from build123d import *

# Parameters (mm, degrees)
EXTRUDE_1_DEPTH          = 2
EXTRUDE_3_DEPTH          = 2
SKETCH_5_W               = 7
SKETCH_5_H               = 7
SKETCH_5_R               = 1.25
EXTRUDE_4_DEPTH          = 7
SKETCH_6_W               = 7
SKETCH_6_H               = 7
SKETCH_6_R               = 1.25
EXTRUDE_5_DEPTH          = 7
CUT_EXTRUDE_1_DEPTH      = 7
CUT_EXTRUDE_1_DEPTH_BACK = 2


with BuildPart() as part:
    # Эскиз1 → Бобышка-Вытянуть1 (new body)
    with BuildSketch(Plane.XY):
        Polygon((-30, 20.5), (-28, 22.5), (4.828427125, 22.5), (12.328427125, 15), (28, 15), (30, 13), (30, -22.5), (-30, -22.5), align=None)
    extrude(amount=EXTRUDE_1_DEPTH)

    # Эскиз4 → Бобышка-Вытянуть3 (add)
    with BuildSketch(Plane(origin=(0, 0, 0), x_dir=(-1, 0, 0), z_dir=(0, 0, -1))):
        Polygon((-27.7, -20.2), (-27.7, 12.7), (-11.375735931, 12.7), (-3.875735931, 20.2), (27.7, 20.2), (27.7, -20.2), align=None)
        Polygon((-25.7, 10.7), (-10.547308807, 10.7), (-3.047308807, 18.2), (25.7, 18.2), (25.7, -18.2), (-25.7, -18.2), align=None, mode=Mode.SUBTRACT)
    extrude(amount=EXTRUDE_3_DEPTH)

    # Эскиз5 → Бобышка-Вытянуть4 (add)
    with BuildSketch(Plane(origin=(27.7, 0, 0), x_dir=(0, 0, -1), z_dir=(1, 0, 0))):
        with Locations((3.5, 9.2)):
            Rectangle(SKETCH_5_W, SKETCH_5_H)
        with Locations((3.5, 9.2)):
            Circle(SKETCH_5_R, mode=Mode.SUBTRACT)
    extrude(amount=-EXTRUDE_4_DEPTH)

    # Эскиз6 → Бобышка-Вытянуть5 (add)
    with BuildSketch(Plane.ZY.offset(27.7)):
        with Locations((-3.5, 16.7)):
            Rectangle(SKETCH_6_W, SKETCH_6_H)
        with Locations((-3.5, 16.7)):
            Circle(SKETCH_6_R, mode=Mode.SUBTRACT)
    extrude(amount=-EXTRUDE_5_DEPTH)

    # Эскиз7 → Вырез-Вытянуть1 (cut, two sides)
    with BuildSketch(Plane(origin=(0, 0, 0), x_dir=(-1, 0, 0), z_dir=(0, 0, -1))) as cut_extrude_1_sk:
        with BuildLine():
            Line((26.5, 7.555), (26.5, -7.525))
            ThreePointArc((26.5, -7.525), (23.5, -10.525), (20.5, -7.525))
            Line((20.5, -7.525), (20.5, 7.555))
            ThreePointArc((20.5, 7.555), (23.5, 10.555), (26.5, 7.555))
        make_face()
    extrude(amount=CUT_EXTRUDE_1_DEPTH, mode=Mode.SUBTRACT)
    extrude(cut_extrude_1_sk.sketch, amount=-CUT_EXTRUDE_1_DEPTH_BACK, mode=Mode.SUBTRACT)


solid = part.part
Part model, mm, in its own coordinate system. A direction names the side the tool comes from. Coordinates: 2 decimals unless noted, no trailing zeros. Loops run counter-clockwise (first coordinate to the right, second up) from the corner with the lowest first, then second, coordinate; pieces in that order, holes last. Notation, with made-up numbers: M 30,35 L 84,35 A24 cw 84,69 Z; hole C -36,-13 d8. An arc over 180 degrees is marked long. Use a Markdown table: item, result. Add a question column.
Q1. Cut at A-A (z = -3.5). Write the cut outline in (x, y), and give its area (3 significant figures).
Q2. Cut at B-B (y = 0.5). Write the cut outline in (x, z).
Q3. Mould opens along X. For faces 6 (the flat face through (-24, 17, -7)), 7 (the flat face through (30, -5, 1)), 8 (the cylindrical face through (-24.59, -10.32, 0.47)) say: +X half, -X half, draft (parallel to the pull), parting line (faces both ways), or undercut.
Q4. Cut at C-C (x = 13). Write the cut outline in (y, z).
Q5. Which spindle directions (+Z, -Z, +X, -X, +Y, -Y) get a long thin tool onto all of the face, cutting with end or side? Do faces 1 (the flat face through (0, 19, -2)), 2 (the flat face through (0, -22.5, 1)), 3 (the cylindrical face through (-24.464, 10.396, 0.472)), 4 (the flat face through (7.678, 16.398, -0.986)), 5 (the flat face through (24, 5.7, -3)). Say none if no direction does.
Q6. Cut at D-D (x = 25). Write the cut outline in (y, z), and give its area (3 significant figures).
Q7. Probe L1, parallel to Y at x = 22.25, z = -3.5; L2, parallel to X at y = 6.5, z = -0.5; L3, parallel to Y at x = 24.5, z = -1. List the from-to ranges inside material, lowest first.
Q8. Pin check, flat tips, straight feed: P1, Ø1, axis at x = 5.5, z = -3, coming from the -Y side; P2, Ø0.6, axis at x = 11.5, z = -1, coming from the -Y side; P3, Ø2, axis at x = 0, y = 1.5, coming from the -Z side; P4, Ø1.6, axis at x = 12.5, z = -1, coming from the +Y side. Stop position of each tip, or through.
Worked out:
| question | item | result |
|---|---|---|
| 1 | outline | M -27.7,13.2 L -20.7,13.2 L -20.7,15.45 L -27.7,15.45 Z; M -27.7,17.95 L -20.7,17.95 L -20.7,20.2 L -27.7,20.2 Z; M 20.7,5.7 L 27.7,5.7 L 27.7,7.95 L 20.7,7.95 Z; M 20.7,10.45 L 27.7,10.45 L 27.7,12.7 L 20.7,12.7 Z |
| 1 | area | 63.0 mm2 |
| 2 | outline | M -30,0 L -27.7,0 L -27.7,-2 L -26.5,-2 L -26.5,2 L -30,2 Z; M -20.5,0 L 25.7,0 L 25.7,-2 L 27.7,-2 L 27.7,0 L 30,0 L 30,2 L -20.5,2 Z |
| 3 | face 6 | draft |
| 3 | face 7 | +X half |
| 3 | face 8 | undercut |
| 4 | outline | M -22.5,0 L -20.2,0 L -20.2,-2 L -18.2,-2 L -18.2,0 L 10.7,0 L 10.7,-2 L 12.7,-2 L 12.7,0 L 15,0 L 15,2 L -22.5,2 Z |
| 5 | face 1 | -Z, +Y, -Y |
| 5 | face 2 | +Z, -Z, +X, -X, -Y |
| 5 | face 3 | +Z, -Z |
| 5 | face 4 | -Z, +X, +Y |
| 5 | face 5 | -Z |
| 6 | outline | M -22.5,0 L -20.2,0 L -20.2,-2 L -18.2,-2 L -18.2,0 L 5.7,0 L 5.7,-7 L 12.7,-7 L 12.7,0 L 15,0 L 15,2 L -22.5,2 Z; hole C 9.2,-3.5 d2.5 |
| 6 | area | 123 mm2 |
| 7 | L1 | y = 5.7 to 7.95, 10.45 to 12.7 |
| 7 | L2 | x = -27.7 to -26.5, 20.7 to 27.7 |
| 7 | L3 | y = -20.2 to -18.2, 5.7 to 12.7 |
| 8 | P1 | passes through |
| 8 | P2 | stops at y = -20.2 |
| 8 | P3 | stops at z = 0 |
| 8 | P4 | stops at y = 12.7 |
